Here's how the part is built. I have some questions about the finished solid (model axes, mm). A direction names the side the tool comes from. Round coordinates to 2 decimals unless told otherwise and drop trailing zeros. Order: outer loops, then holes, each group sorted by start corner. A loop starts at its lowest first (then second) coordinate and runs counter-clockwise, first axis right, second up. Notation, with made-up numbers: (-35, 5.5) - (-25, 5.5) arc R23 ccw to (-25, 18.5) - close; hole circle Ø8 at (31, 82.25). An arc over 180 degrees is marked (long way). Answer as a JSON object with one key per item and string values.
```python
from build123d import *

# Parameters (mm, degrees)
CHAMFER1_SIZE       = 0.05
SKETCH3_R           = 1.5
BOSS_EXTRUDE1_DEPTH = 2


with BuildPart() as part:
    # Sketch1 → Revolve1 (revolve)
    with BuildSketch(Plane.XY):
        with BuildLine():
            Line((0, 0), (1.5, 0))
            Line((1.5, 0), (1.5, 11))
            ThreePointArc((1.5, 11), (2.897777479, 14.374533347), (0, 16.598076211))
            Line((0, 16.598076211), (0, 0))
        make_face()
    revolve(axis=Axis((0, 0, 0), (0, 1, 0)))

    # Chamfer1
    chamfer1_edges = [part.edges().sort_by_distance(p)[0] for p in [
        (-1.5, 0, 0),
    ]]
    chamfer(chamfer1_edges, length=CHAMFER1_SIZE)

    # Sketch3 → Boss-Extrude1 (add)
    with BuildSketch(Plane(origin=(0, 7.5, 0), x_dir=(1, 0, 0), z_dir=(0, 1, 0))):
        Polygon((3, 1.732050808), (0, 3.464101615), (-3, 1.732050808), (-3, -1.732050808), (0, -3.464101615), (3, -1.732050808), align=None)
        Circle(SKETCH3_R, mode=Mode.SUBTRACT)
    extrude(amount=BOSS_EXTRUDE1_DEPTH)


solid = part.part
```
1. Imagine slicing it at D-D (y = 6.75). List the corners of the cut face in (x, z) for me.
Responses:
{"outline": "circle Ø3 at (0, 0)"}
2. If I drill on L1, parallel to X at y = 10.25, z = 0; L2, parallel to Y at x = 2.75, z = 1.5; L3, parallel to Y at x = -2.25, z = -0.25, over which ranges is the centre line in solid material (lowest first)? Write a range as [from, to].
Responses:
{"L1": "[-1.5, 1.5]", "L2": "[7.5, 9.5]", "L3": "[7.5, 9.5], [11.63, 15.57]"}
3. Imagine slicing it at C-C (z = -2.25). List the corners of the cut face in (x, y) for me.
Responses:
{"outline": "(-2.1, 7.5) - (2.1, 7.5) - (2.1, 9.5) - (-2.1, 9.5) - close; circle Ø3.97 at (0, 13.6)"}
4. Imagine slicing it at B-B (x = 1.75). List the corners of the cut face in (y, z) for me.
Responses:
{"outline": "(7.5, -2.45) - (9.5, -2.45) - (9.5, 2.45) - (7.5, 2.45) - close; circle Ø4.87 at (13.6, 0)"}
5. For P1, Ø1, axis at x = 0, y = 14.5, coming from the +Z side, with a flat end and sliding along its axis, tell me the tip position at first contact or that it passes through.
Responses:
{"P1": "z = 2.97"}
6. Thinking about a two-plate mould opening in Y: for faces 4 (the face through (-1.5, 8.5, 2.6)), 5 (the face through (-1.5, 10.26, -0.07)), 6 (the face through (0, 0, 0)), which applies, pulls with the +Y half, pulls with the -Y half, needs draft (parallel to the pull), parting line crosses it, or undercut?
Responses:
{"face 4": "needs draft", "face 5": "undercut", "face 6": "pulls with the -Y half"}
7. Imagine slicing it at A-A (z = 0). List the corners of the cut face in (x, y) for me.
Responses:
{"outline": "(-3, 7.5) - (-1.5, 7.5) - (-1.5, 0.05) - (-1.45, 0) - (1.45, 0) - (1.5, 0.05) - (1.5, 7.5) - (3, 7.5) - (3, 9.5) - (1.5, 9.5) - (1.5, 11) arc R3 ccw (long way) to (-1.5, 11) - (-1.5, 9.5) - (-3, 9.5) - close"}
8. For faces 1 (the face through (1.5, 8.5, 2.6)), 2 (the face through (-0.7, 9.5, 1.5)), 3 (the face through (-0.7, 7.5, 1.5)), which set-ups out of +Z, -Z, +X, -X, +Y, -Y let a thin tool reach every point of the face, with its end or its side?
Responses:
{"face 1": "+Z, +X, +Y, -Y", "face 2": "none", "face 3": "-Y"}
